Geometry: see drawing. Coordinates: mm, zero at the bounding-box minimum. Give positions to 0.01 mm unless a question says otherwise; leave off trailing zeros. Loops run counter-clockwise (first coordinate to the right, second up) from the corner with the lowest first, then second, coordinate; pieces in that order, holes last. Notation, with made-up numbers: (-32, 48.5) -> (-16, 48.5) arc R22 ccw to (-16, 59.5) -> close; hole circle Ø5 at (27.25, 39.25). An arc over 180 degrees is marked (long way). Answer in a Markdown table with one row per item. Add a question column.
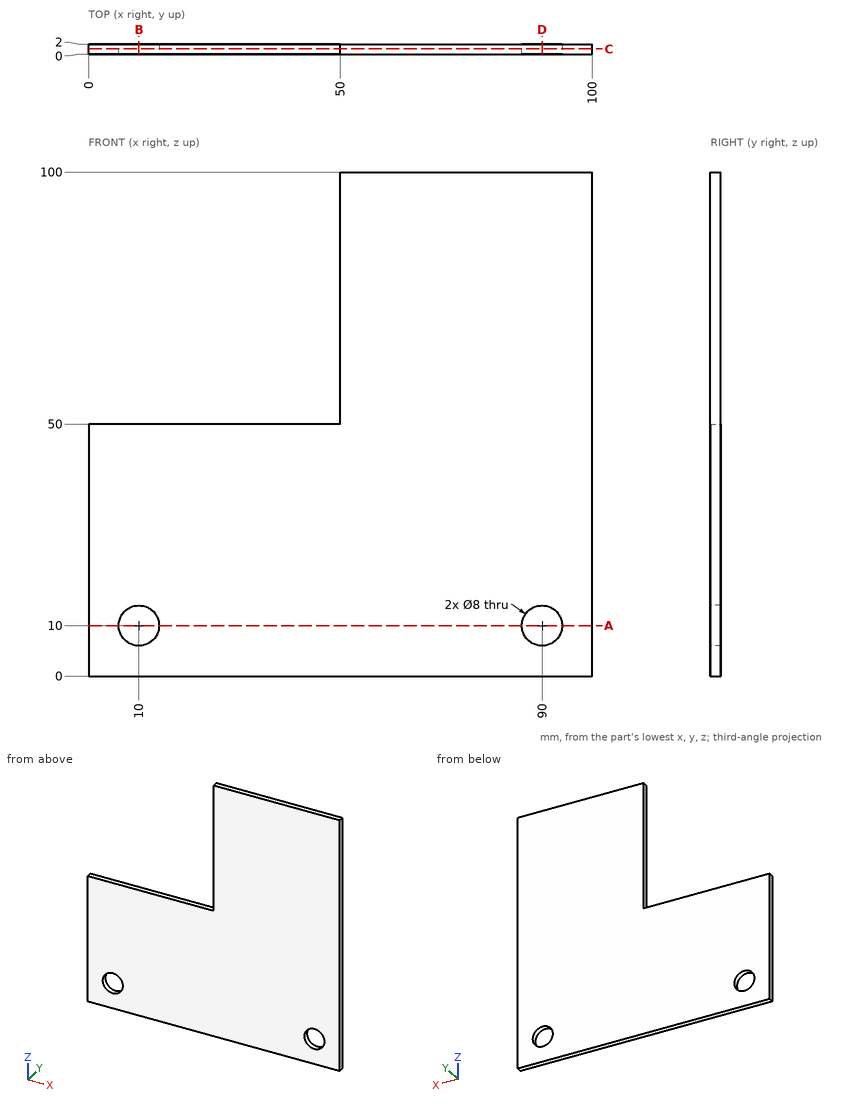
1) Material intervals for line 1 along Z through (x, y) = (10, 1.55); line 2 along Z through (x, y) = (90, 0.9); line 3 along X through (y, z) = (1, 68.5), sorted ascending.
2) Pin query (flat end, axial travel): pin 1 (1 mm diameter, centred on x = 13.5, y = 0.5, fed in from +Z). Return the tip coordinate at first contact, or that it passes through.
3) Section C-C on y = 1.05. Output: boundary loops of the cut face in (x, z), and give its area (3 significant figures).
4) Section D-D on x = 90. Output: boundary loops of the cut face in (y, z), and give its area (3 significant figures).
5) Section A-A on z = 10. Output: boundary loops of the cut face in (x, y).
6) Section B-B on x = 10. Output: boundary loops of the cut face in (y, z).
Working result:
| question | item | result |
|---|---|---|
| 1 | line 1 | z = 0 to 6, 14 to 50 |
| 1 | line 2 | z = 0 to 6, 14 to 100 |
| 1 | line 3 | x = 50 to 100 |
| 2 | pin 1 | stops at z = 50 |
| 3 | outline | (0, 0) -> (100, 0) -> (100, 100) -> (50, 100) -> (50, 50) -> (0, 50) -> close; hole circle Ø8 at (10, 10); hole circle Ø8 at (90, 10) |
| 3 | area | 7,400 mm2 |
| 4 | outline | (0, 0) -> (2, 0) -> (2, 6) -> (0, 6) -> close; (0, 14) -> (2, 14) -> (2, 100) -> (0, 100) -> close |
| 4 | area | 184 mm2 |
| 5 | outline | (0, 0) -> (6, 0) -> (6, 2) -> (0, 2) -> close; (14, 0) -> (86, 0) -> (86, 2) -> (14, 2) -> close; (94, 0) -> (100, 0) -> (100, 2) -> (94, 2) -> close |
| 6 | outline | (0, 0) -> (2, 0) -> (2, 6) -> (0, 6) -> close; (0, 14) -> (2, 14) -> (2, 50) -> (0, 50) -> close |
